from build123d import *

# Parameters (mm, degrees)
BOSS_EXTRUDE1_DEPTH          = 3.175
SKETCH6_W                    = 38.1
SKETCH6_H                    = 50.8
BOSS_EXTRUDE3_DEPTH          = 12.7
FILLET1_R                    = 7.62
SKETCH2_R                    = 2.15265
MOUNTINGHOLESM4_DEPTH        = 3.175
SKETCH5_R                    = 12.7
HOLEFOR25MMOUTCROPPING_DEPTH = 3.175
SKETCH7_R                    = 2.15265
CUT_EXTRUDE4_DEPTH           = 15.875


with BuildPart() as part:
    # Sketch1 → Boss-Extrude1 (new body)
    with BuildSketch(Plane(origin=(0, 0, 0), x_dir=(1, 0, 0), z_dir=(0, 1, 0))):
        Polygon((50.8, 25.4), (63.5, 25.4), (63.5, -25.4), (50.8, -25.4), (0, -25.4), (-38.1, -25.4), (-38.1, 25.4), (0, 25.4), align=None)
    extrude(amount=BOSS_EXTRUDE1_DEPTH)

    # Sketch6 → Boss-Extrude3 (add)
    with BuildSketch(Plane(origin=(0, 3.175, 0), x_dir=(1, 0, 0), z_dir=(0, 1, 0))):
        with Locations((-19.05, 0)):
            Rectangle(SKETCH6_W, SKETCH6_H)
    extrude(amount=BOSS_EXTRUDE3_DEPTH)

    # Fillet1
    fillet1_edges = [part.edges().sort_by_distance(p)[0] for p in [
        (0, 3.175, 0),
    ]]
    fillet(fillet1_edges, radius=FILLET1_R)

    # Sketch2 → MountingHolesM4 (cut)
    with BuildSketch(Plane(origin=(0, 3.175, 0), x_dir=(1, 0, 0), z_dir=(0, 1, 0))):
        with Locations((50.474368671, 12.374368671)):
            Circle(SKETCH2_R)
        with Locations((50.474368671, -12.374368671)):
            Circle(SKETCH2_R)
        with Locations((25.725631329, -12.374368671)):
            Circle(SKETCH2_R)
        with Locations((25.725631329, 12.374368671)):
            Circle(SKETCH2_R)
    extrude(amount=-MOUNTINGHOLESM4_DEPTH, mode=Mode.SUBTRACT)

    # Sketch5 → HoleFor25mmOutCropping (cut)
    with BuildSketch(Plane(origin=(0, 3.175, 0), x_dir=(1, 0, 0), z_dir=(0, 1, 0))):
        with Locations((38.1, 0)):
            Circle(SKETCH5_R)
    extrude(amount=-HOLEFOR25MMOUTCROPPING_DEPTH, mode=Mode.SUBTRACT)

    # Sketch7 → Cut-Extrude4 (cut)
    with BuildSketch(Plane.XZ):
        with Locations((-9.525, -12.7)):
            Circle(SKETCH7_R)
        with Locations((-28.575, -12.7)):
            Circle(SKETCH7_R)
        with Locations((-9.525, 12.7)):
            Circle(SKETCH7_R)
        with Locations((-28.575, 12.7)):
            Circle(SKETCH7_R)
    extrude(amount=-CUT_EXTRUDE4_DEPTH, mode=Mode.SUBTRACT)


solid = part.part
Part model, mm, in its own coordinate system. A direction names the side the tool comes from. Coordinates: 2 decimals unless noted, no trailing zeros. Order: outer loops, then holes, each group sorted by start corner. A loop starts at its lowest first (then second) coordinate and runs counter-clockwise, first axis right, second up. Notation, with made-up numbers: M -1,-7 L 47,-7 A38 cw 47,32 Z; hole C 80,21 d10. An arc over 180 degrees is marked long. Use a Markdown table: item, result.
(1) Cut at C-C on y = 12.75. Write the cut outline in (x, z) (3 decimals).
A:
| item | result |
|---|---|
| outline | M -38.1,-25.4 L 0,-25.4 L 0,25.4 L -38.1,25.4 Z; hole C -28.575,-12.7 d4.305; hole C -28.575,12.7 d4.305; hole C -9.525,-12.7 d4.305; hole C -9.525,12.7 d4.305 |
(2) Cut at D-D on z = -7. Write the cut outline in (x, y) (3 decimals), then the cut area to 3 significant figures.
A:
| item | result |
|---|---|
| outline | M -38.1,0 L 27.503,0 L 27.503,3.175 L 7.62,3.175 A7.62 cw 0,10.795 L 0,15.875 L -38.1,15.875 Z; M 48.697,0 L 63.5,0 L 63.5,3.175 L 48.697,3.175 Z |
| area | 752 mm^2 |
(3) Cut at A-A on x = 38.1. Write the cut outline in (y, z) (3 decimals), then the cut area to 3 significant figures.
A:
| item | result |
|---|---|
| outline | M 0,-25.4 L 3.175,-25.4 L 3.175,-12.7 L 0,-12.7 Z; M 0,12.7 L 3.175,12.7 L 3.175,25.4 L 0,25.4 Z |
| area | 80.6 mm^2 |
(4) Pull direction Z, two halves, no side cores. Call faces 3 (the cylindrical face through (52.53, 1.61, -13.02)), 4 (the flat face through (-38.1, 8, 0)), 5 (the flat face through (-11, 6, 25.4)): released by +Z, released by -Z, zero draft, split by the parting line, or undercut.
A:
| item | result |
|---|---|
| face 3 | undercut |
| face 4 | zero draft |
| face 5 | released by +Z |
(5) Tool access for faces 1 (the flat face through (24, 3.175, 0)), 2 (the flat face through (-19, 15.875, 0)): list every direction of +Z, -Z, +X, -X, +Y, -Y with a clear straight run to the whole face (end or side of a thin tool).
A:
| item | result |
|---|---|
| face 1 | +Z, -Z, +X, +Y |
| face 2 | +Z, -Z, +X, -X, +Y |
(6) Flat gauge pins, fed straight in: pin 1 (10 mm diameter, centred on x = 45.5, z = 15.5, fed in from +Y) (3 decimals); pin 2 (1.5 mm diameter, centred on y = 14, z = -10, fed in from +X). Where does each tip first touch, or does it go through?
A:
| item | result |
|---|---|
| pin 1 | stops at y = 3.175 |
| pin 2 | stops at x = 0 |
(7) Cut at B-B on z = -17. Write the cut outline in (x, y) (3 decimals).
A:
| item | result |
|---|---|
| outline | M -38.1,0 L 63.5,0 L 63.5,3.175 L 7.62,3.175 A7.62 cw 0,10.795 L 0,15.875 L -38.1,15.875 Z |
(8) Probe L1, parallel to Z at x = -28.5, y = 7.75; L2, parallel to X at y = 6.5, z = 14; L3, parallel to Y at x = 51.5, z = -4 (3 decimals). List the from-to ranges inside material, lowest first.
A:
| item | result |
|---|---|
| L1 | z = -25.4 to -14.85, -10.55 to 10.55, 14.85 to 25.4 |
| L2 | x = -38.1 to -30.29, -26.86 to -11.24, -7.81 to 1.33 |
| L3 | y = 0 to 3.175 |
